from build123d import *

# Parameters (mm, degrees)
F0_R      = 7.9822757018
F1_DEPTH  = 25.4
F2_W      = 31.536786817
F2_H      = 54.3133597821
F3_DEPTH  = 38.1
F5_DEPTH  = 35.56
F7_DEPTH  = 33.02
F9_DEPTH  = 33.02
F10_R     = 3.1631900108
F11_DEPTH = 33.02
F12_R     = 3.540896841
F13_DEPTH = 33.02


with BuildPart() as f1:
    # F0 (on Top) → F1 (new body)
    with BuildSketch(Plane.XY):
        with BuildLine():
            Line((24.3826080114, -38.690969348), (24.3826080114, 39.5669899881))
            ThreePointArc((24.3826080114, 39.5669899881), (0.2920059487, 63.6575920507), (-23.7985961139, 39.5669899881))
            Line((-23.7985961139, 39.5669899881), (-23.7985961139, -38.690969348))
            ThreePointArc((-23.7985961139, -38.690969348), (0.2920059487, -62.7815714106), (24.3826080114, -38.690969348))
        make_face()
        with Locations((0.2920059487, -38.690969348)):
            Circle(F0_R, mode=Mode.SUBTRACT)
        with Locations((0.2920059487, 39.5669899881)):
            Circle(F0_R, mode=Mode.SUBTRACT)
    extrude(amount=F1_DEPTH)

    # F2 (on face) → F3 (join)
    with BuildSketch(Plane.XY.offset(25.4)):
        with Locations((0.4380107857, 0.1460043713)):
            Rectangle(F2_W, F2_H)
    extrude(amount=F3_DEPTH)

    # F4 (on face) → F5 (cut)
    with BuildSketch(Plane.YZ.offset(16.2064041942)):
        with BuildLine():
            Line((13.6914392933, 48.9439629018), (13.6914392933, 63.5))
            Line((13.6914392933, 63.5), (-13.0694909021, 63.5))
            Line((-13.0694909021, 63.5), (-13.0694909021, 48.9439629018))
            ThreePointArc((-13.0694909021, 48.9439629018), (0.3109741956, 35.5634978041), (13.6914392933, 48.9439629018))
        make_face()
    extrude(amount=-F5_DEPTH, mode=Mode.SUBTRACT)

    # F6 (on face) → F7 (cut)
    with BuildSketch(Plane.XZ.offset(27.0106755197)):
        with BuildLine():
            ThreePointArc((-15.3303826228, 51.122944802), (-0.0918545456, 63.4173583867), (16.2064041942, 52.5669157505))
            Line((16.2064041942, 52.5669157505), (16.2064041942, 63.5))
            Line((16.2064041942, 63.5), (-15.3303826228, 63.5))
            Line((-15.3303826228, 63.5), (-15.3303826228, 51.122944802))
        make_face()
    extrude(amount=-F7_DEPTH, mode=Mode.SUBTRACT)

    # F8 (on face) → F9 (cut)
    with BuildSketch(Plane(origin=(0, 27.3026842624, 0), x_dir=(-1, 0, 0), z_dir=(0, 1, 0))):
        with BuildLine():
            ThreePointArc((-16.2064041942, 52.8267547488), (-0.2710597584, 62.9963273127), (15.3303826228, 52.3215718567))
            Line((15.3303826228, 52.3215718567), (15.3303826228, 63.5))
            Line((15.3303826228, 63.5), (-16.2064041942, 63.5))
            Line((-16.2064041942, 63.5), (-16.2064041942, 52.8267547488))
        make_face()
    extrude(amount=-F9_DEPTH, mode=Mode.SUBTRACT)

    # F10 (on face) → F11 (cut)
    with BuildSketch(Plane(origin=(0, 27.3026842624, 0), x_dir=(-1, 0, 0), z_dir=(0, 1, 0))):
        with Locations((0, 55.5282048881)):
            Circle(F10_R)
    extrude(amount=-F11_DEPTH, mode=Mode.SUBTRACT)

    # F12 (on face) → F13 (cut)
    with BuildSketch(Plane.XZ.offset(27.0106755197)):
        with Locations((0.4380107857, 54.8420138657)):
            Circle(F12_R)
    extrude(amount=-F13_DEPTH, mode=Mode.SUBTRACT)


solid = f1.part
Work out the finished part from the listing and answer in its coordinate system (mm). A direction names the side the tool comes from. Coordinates: 2 decimals unless noted, no trailing zeros. Loops run counter-clockwise (first coordinate to the right, second up) from the corner with the lowest first, then second, coordinate; pieces in that order, holes last. Notation, with made-up numbers: M 39.5,-20 L 47.5,-20 A27 ccw 47.5,9 Z; hole C 49,-17 d9. An arc over 180 degrees is marked long. Answer in a Markdown table with one row per item. Add a question column.
1. The mould has two halves that part along Y. Classify faces 1 (the flat face through (-16, 1, 25.4)), 2 (the flat face through (0, -27.011, 44)), 3 (the cylindrical face through (-0.747, -30.777, 12.522)): pulls with the +Y half, pulls with the -Y half, needs draft (parallel to the pull), parting line crosses it, or undercut.
2. A tool of negligible diameter and unlimited length cuts with its end or side. For faces 4 (the cylindrical face through (0.6, 20.6, 63)), 5 (the flat face through (4.2, -13.069, 54.7)), 6 (the cylindrical face through (0.412, 20.592, 58.664)), 7 (the cylindrical face through (-0.4, -20.1, 63.4)), from which of +Z, -Z, +X, -X, +Y, -Y can it reach the whole face along a straight path? Write none if from no direction.
3. Find section A-A, the plane z = 42. Write down the section's boundary in (x, y).
4. Find section B-B, the plane y = -42. Write down the section's boundary in (x, z), then the cut area to 3 significant figures.
5. Find section C-C, the plane x = 0. Write down the section's boundary in (y, z).
6. Find section D-D, the plane y = 17.5. Write down the section's boundary in (x, z), then the cut area to 3 significant figures.
7. Consider L1, parallel to Y at x = -1.5, z = 51.5; L2, parallel to Z at x = 0.5, y = -24.5; L3, parallel to Z at x = 0, y = 20. Determine where each line is inside the solid, lowest interval first.
8. Flat-ended cylindrical pins translate along their axes: P1, Ø11.5, axis at x = 0.44, z = 54.84, coming from the -Y side; P2, Ø2, axis at x = -8.5, z = 38.5, coming from the +Y side; P3, Ø3, axis at y = 14, z = 51.5, coming from the -X side; P4, Ø14.5, axis at x = 0.29, y = 39.57, coming from the -Z side. Find the tip coordinate at first contact, or state that the pin passes through.
Reported:
| question | item | result |
|---|---|---|
| 1 | face 1 | needs draft |
| 1 | face 2 | pulls with the -Y half |
| 1 | face 3 | undercut |
| 2 | face 4 | +Z, +Y |
| 2 | face 5 | +Z, +X, -X |
| 2 | face 6 | +Y |
| 2 | face 7 | +Z, -Y |
| 3 | outline | M -15.33,-27.01 L 16.21,-27.01 L 16.21,-11.13 L -15.33,-11.13 Z; M -15.33,11.75 L 16.21,11.75 L 16.21,27.3 L -15.33,27.3 Z |
| 4 | outline | M -23.57,0 L -6.97,0 L -6.97,25.4 L -23.57,25.4 Z; M 7.56,0 L 24.15,0 L 24.15,25.4 L 7.56,25.4 Z |
| 4 | area | 843 mm^2 |
| 5 | outline | M -62.78,0 L -46.67,0 L -46.67,25.4 L -62.78,25.4 Z; M -30.71,0 L 31.59,0 L 31.59,25.4 L 27.3,25.4 L 27.3,52.37 L 13.69,52.37 L 13.69,48.94 A13.38 cw -13.07,48.94 L -13.07,51.33 L -27.01,51.33 L -27.01,25.4 L -30.71,25.4 Z; M -27.01,58.36 L -13.07,58.36 L -13.07,63.42 L -27.01,63.42 Z; M 13.69,58.69 L 27.3,58.69 L 27.3,62.99 L 13.69,62.99 Z; M 47.54,0 L 63.66,0 L 63.66,25.4 L 47.54,25.4 Z |
| 6 | outline | M -23.8,0 L 24.38,0 L 24.38,25.4 L 16.21,25.4 L 16.21,52.83 A17.14 ccw -15.33,52.32 L -15.33,25.4 L -23.8,25.4 Z; hole C 0,55.53 d6.33 |
| 6 | area | 2,290 mm^2 |
| 7 | L1 | y = -27.01 to -13.07, 13.69 to 27.3 |
| 7 | L2 | z = 0 to 51.3, 58.38 to 63.43 |
| 7 | L3 | z = 0 to 52.37, 58.69 to 62.99 |
| 8 | P1 | stops at y = -27.01 |
| 8 | P2 | stops at y = 27.3 |
| 8 | P3 | stops at x = -15.33 |
| 8 | P4 | passes through |
